Autodesk Inventor part; units mm, degrees
ref_plane "Plano de trabajo1" through (0, 0, -347.5) normal (0, 0, 1) x (1, 0, 0)
ref_plane "YZ Plane" through (0, 0, 0) normal (1, 0, 0) x (0, 1, 0)
ref_plane "XZ Plane" through (0, 0, 0) normal (0, 1, 0) x (-1, 0, 0)
sketch "Boceto1" plane through (0, 0, 0) normal (0, 0, 1) x (1, 0, 0)
  line L0 (28.1307, 40.0149) -> (1.9307, 40.0149)
  line L1 (1.9307, 41.4149) -> (28.1307, 41.4149)
  line L2 (0.0307, -0.1851) -> (0.0307, 51.6749)
  line L3 (24.8307, 55.8149) -> (24.8307, 54.1749)
  line L4 (28.6307, 54.4149) -> (28.6307, 47.9149)
  line L5 (28.6307, 46.5149) -> (24.8307, 46.5149)
  line L6 (24.8307, 46.5149) -> (24.8307, 48.1549)
  line L7 (26.2307, 47.9149) -> (28.6307, 47.9149)
  line L8 (26.2307, 49.1649) -> (25.5249, 49.1649)
  line L9 (25.5249, 49.1649) -> (24.8307, 48.1549)
  line L10 (26.2307, 53.1649) -> (25.5249, 53.1649)
  line L11 (1.4307, 41.9149) -> (1.4307, 48.9149)
  line L12 (1.4307, 48.9149) -> (2.9307, 48.9149)
  line L13 (2.9307, 48.9149) -> (2.9307, 51.6749)
  line L14 (4.1707, 55.8149) -> (10.8307, 55.8149)
  line L15 (9.3926, 54.4149) -> (5.6707, 54.4149)
  line L16 (10.8307, 55.8149) -> (10.8307, 53.3149)
  line L17 (10.8307, 53.3149) -> (10.1207, 53.3149)
  line L18 (10.1207, 53.3149) -> (9.3926, 54.4149)
  line L19 (26.2307, 54.4149) -> (28.6307, 54.4149)
  arc A0 (5.6707, 54.4149) -> (2.9307, 51.6749) centre (5.6707, 51.6749) ccw
  arc A1 (4.1707, 55.8149) -> (0.0307, 51.6749) centre (4.1707, 51.6749) ccw
  line L20 (24.8307, 54.1749) -> (25.5249, 53.1649)
  line L21 (26.2307, 54.4149) -> (26.2307, 53.1649)
  line L22 (26.2307, 47.9149) -> (26.2307, 49.1649)
  arc A2 (1.9307, 40.0149) -> (1.4307, 39.5149) centre (1.9307, 39.5149) ccw
  arc A3 (28.6307, 39.5149) -> (28.1307, 40.0149) centre (28.1307, 39.5149) ccw
  arc A4 (28.1307, 41.4149) -> (28.6307, 41.9149) centre (28.1307, 41.9149) ccw
  arc A5 (1.4307, 41.9149) -> (1.9307, 41.4149) centre (1.9307, 41.9149) ccw
  line L23 (30.0307, 55.8149) -> (24.8307, 55.8149)
  line L24 (28.6307, 41.9149) -> (28.6307, 46.5149)
  line L25 (30.0307, 55.8149) -> (30.0307, -0.1851)
  line L26 (1.4307, 29.0149) -> (28.6307, 29.0149)
  line L27 (1.4307, 27.6149) -> (28.6307, 27.6149)
  line L28 (1.4307, 39.5149) -> (1.4307, 29.0149)
  line L29 (1.4307, 27.6149) -> (1.4307, 1.2149)
  line L30 (28.6307, 1.2149) -> (28.6307, 27.6149)
  line L31 (28.6307, 29.0149) -> (28.6307, 39.5149)
  line L32 (28.6307, 39.5149) -> (28.6307, 29.0149)
  line L33 (28.6307, 27.6149) -> (28.6307, 1.2149)
  line L34 (4.5307, 5.9149) -> (6.8307, 5.9149)
  line L35 (7.8307, 4.9149) -> (7.8307, 2.5149)
  line L36 (7.8307, 2.5149) -> (6.4307, 2.5149)
  line L37 (6.4307, 2.5149) -> (6.4307, 4.5149)
  line L38 (6.4307, 4.5149) -> (4.9307, 4.5149)
  line L39 (4.9307, 4.5149) -> (4.9307, -3.4851)
  line L40 (4.9307, -3.4851) -> (6.4307, -3.4851)
  line L41 (6.4307, -3.4851) -> (6.4307, -1.4851)
  line L42 (6.4307, -1.4851) -> (7.8307, -1.4851)
  line L43 (7.8307, -1.4851) -> (7.8307, -3.8851)
  line L44 (6.8307, -4.8851) -> (3.5307, -4.8851)
  line L45 (3.5307, -4.8851) -> (3.5307, -0.1851)
  arc A6 (7.8307, 4.9149) -> (6.8307, 5.9149) centre (6.8307, 4.9149) ccw
  arc A7 (4.5307, 5.9149) -> (3.5307, 4.9149) centre (4.5307, 4.9149) ccw
  arc A8 (6.8307, -4.8851) -> (7.8307, -3.8851) centre (6.8307, -3.8851) ccw
  line L46 (3.5307, 1.2149) -> (1.4307, 1.2149)
  line L47 (3.5307, -0.1851) -> (0.0307, -0.1851)
  line L48 (3.5307, 1.2149) -> (3.5307, 4.9149)
  line L49 (25.5307, 5.9149) -> (23.2307, 5.9149)
  line L50 (22.2307, 4.9149) -> (22.2307, 2.5149)
  line L51 (22.2307, 2.5149) -> (23.6307, 2.5149)
  line L52 (23.6307, 2.5149) -> (23.6307, 4.5149)
  line L53 (23.6307, 4.5149) -> (25.1307, 4.5149)
  line L54 (25.1307, 4.5149) -> (25.1307, -3.4851)
  line L55 (25.1307, -3.4851) -> (23.6307, -3.4851)
  line L56 (23.6307, -3.4851) -> (23.6307, -1.4851)
  line L57 (23.6307, -1.4851) -> (22.2307, -1.4851)
  line L58 (22.2307, -1.4851) -> (22.2307, -3.8851)
  line L59 (23.2307, -4.8851) -> (26.5307, -4.8851)
  line L60 (26.5307, -4.8851) -> (26.5307, -0.1851)
  arc A9 (23.2307, 5.9149) -> (22.2307, 4.9149) centre (23.2307, 4.9149) ccw
  arc A10 (26.5307, 4.9149) -> (25.5307, 5.9149) centre (25.5307, 4.9149) ccw
  arc A11 (22.2307, -3.8851) -> (23.2307, -4.8851) centre (23.2307, -3.8851) ccw
  line L61 (26.5307, 1.2149) -> (28.6307, 1.2149)
  line L62 (26.5307, -0.1851) -> (30.0307, -0.1851)
  line L63 (26.5307, 1.2149) -> (26.5307, 4.9149)
  point P0 (28.6307, 51.1649)
  point P1 (0.0307, 0.7149)
  point P2 (4.9307, 0.5149)
  point P3 (25.1307, 0.5149)
  dimension "d31" = 1.4
  dimension "d42" = 2.5
  dimension "d43" = 0.71
  dimension "d45" = 2.9
  dimension "d47" = 33.5
  dimension "d48" = 7.5
  dimension "d51" = 2.74
  dimension "d59" = 6.9
  dimension "d60" = 1.4
  dimension "d78" = 6.5
  dimension "d84" = 1.4
  dimension "d85" = 1.4
  dimension "d88" = 2.4
  dimension "d95" = 6.02
  dimension "d99" = 111
  dimension "d100" = 2.4
  dimension "d108" = 4
  dimension "d109" = 0.7058
  dimension "d110" = 0.7058
  dimension "d143" = 1.4
  dimension "d147" = 1.4
  dimension "d148" = 30
  dimension "d149" = 1.4
  dimension "d150" = 14
  dimension "d151" = 27.2
  dimension "d152" = 14.4
  dimension "d153" = 1.4
  dimension "d154" = 11
  dimension "d155" = 1.4
  dimension "d156" = 1.4
  dimension "d157" = 1.4
  dimension "d158" = 1.4
  dimension "d162" = 60.7
  dimension "d163" = 10.8
  dimension "d164" = 8
  dimension "d165" = 2
  dimension "d166" = 4
  dimension "d167" = 1.5
  dimension "d168" = 7.8
  dimension "d169" = 1
  dimension "d172" = 1.4
  dimension "d173" = 4.7
  dimension "d175" = 56
  dimension "d176" = 13.8
  dimension "d177" = 14.4
  dimension "d180" = 1.5
  dimension "d181" = 4.14
  dimension "d182" = 10.8
  dimension "d183" = 14.4
  dimension "d184" = 0.5
  dimension "d187" = 3.5
  dimension "d188" = 4.9
  dimension "d189" = 6.4
  dimension "d190" = 7.8
  dimension "d191" = 26.5
  dimension "d193" = 54.6
  dimension "d195" = 3.5
  dimension "d196" = 4.9
  dimension "d197" = 53.9
  dimension "d198" = 53.7
  dimension "d202" = 2
  dimension "d203" = 3.01
  dimension "d204" = 2
  dimension "d205" = 9.3
extrude "Extrusión1" add sketch "Boceto1" against normal blind 695
ref_plane "Plano de trabajo1" through (0, 0, -347.5) normal (0, 0, 1) x (1, 0, 0)
sketch "Boceto2" plane through (30.0307, -0.1851, 0) normal (1, 0, 0) x (0, 0, -1)
  line L0 (0, -4.7) -> (0, 0)
  line L1 (0, -4.7) -> (695, -4.7)
  line L2 (695, 0) -> (695, -4.7)
  line L3 (0, 0) -> (695, 0)
  line L4 (0, 0) -> (0, 56)
  line L5 (0, 0) -> (695, 0)
  line L6 (695, 56) -> (695, 0)
  line L7 (0, 56) -> (695, 56)
  line L8 (0, -4.7) -> (60.7, 56)
  line L9 (0, 56) -> (60.7, 56)
  line L10 (0, 56) -> (0, -4.7)
  point P0 (0, 0.1851)
  point P1 (0, 0)
  dimension "d201" = 45
extrude "Extrusión2" cut sketch "Boceto2" against normal through all contours L0 L3 L8 | L4 L7 L8 L3
mirror "Simetría1" about plane through (0, 0, -347.5) normal (0, 0, 1) of "Extrusión2"
ref_plane "Plano de trabajo2" through (15.0307, -0.1851, -4.7) normal (1, 0, 0) x (0, 0, -1)
properties part number "SP40-10 HOJA CORREDERA 695 mm" material "Aluminio"
Model file for the job. Use its own axes, mm. A direction names the side the tool comes from. Coordinates: 2 decimals unless noted, no trailing zeros. Write each loop counter-clockwise with the first axis right and the second up, starting at its lowest first coordinate (ties: lowest second). Pieces come first, ordered by that corner, then holes. Notation, with made-up numbers: (-26.5, 13.25) - (4.5, 13.25) arc R16 ccw to (4.5, 20.25) - close; hole circle Ø6 at (77.25, 61). An arc over 180 degrees is marked (long way). One line per question, with ' | ' between items. Start each with the question number.
Q1. Pin check, flat tips, straight feed: pin 1 (3 mm diameter, centred on x = 11.5, z = -129.5, fed in from +Y); pin 2 (2 mm diameter, centred on y = -2.5, z = -354.5, fed in from +X); pin 3 (1.7 mm diameter, centred on x = 2, z = -510, fed in from +Y). Stop position of each tip, or through.
Q2. Cut at A-A, the plane x = 17.5. List the corners of the cut face in (y, z), then the cut area to 3 significant figures.
Q3. 3-axis set-ups, long thin cutter, end or side, ignore diameter. For faces 5 (the face through (28.631, 34, -343)), 6 (the face through (0.656, 27.571, -32.457)): which of +Z, -Z, +X, -X, +Y, -Y reach the whole face in a straight line?
Q4. Pull direction X, two halves, no side cores. Call faces 1 (the face through (30.031, 28, -343)), 2 (the face through (13.99, 27.855, -662.26)), 3 (the face through (28.631, 14, -343)), 4 (the face through (0.031, 25, -343)): pulls with the +X half, pulls with the -X half, needs draft (parallel to the pull), parting line crosses it, or undercut.
Q5. Drill centre lines: line 1 (X direction, y = 5, z = -119); line 2 (Y direction, x = 9, z = -316); line 3 (Y direction, x = 27.75, z = -603.5). Where is each one in solid material? Low to high. Write a range as [from, to].
Answer below:
1) pin 1: y = 55.81 | pin 2: x = 26.53 | pin 3: y = 55.6
2) outline: (27.61, -662.5) - (29.01, -661.1) - (29.01, -33.9) - (27.61, -32.5) - close; (40.01, -650.1) - (41.41, -648.7) - (41.41, -46.3) - (40.01, -44.9) - close | area: 1,730 mm^2
3) face 5: +Z, -Z | face 6: +Z, +X, -X, +Y
4) face 1: pulls with the +X half | face 2: needs draft | face 3: undercut | face 4: pulls with the -X half
5) line 1: [0.03, 1.43], [3.53, 7.83], [22.23, 26.53], [28.63, 30.03] | line 2: [27.61, 29.01], [40.01, 41.41], [54.41, 55.81] | line 3: [-0.19, 1.21], [27.61, 29.01], [40.01, 41.41], [46.51, 47.91], [54.41, 55.81]
